For this review, take the finished solid that the model builds, in its own axes (mm). A direction names the side the tool comes from. Give positions to 0.01 mm unless a question says otherwise; leave off trailing zeros. Write each loop counter-clockwise with the first axis right and the second up, starting at its lowest first coordinate (ties: lowest second). Pieces come first, ordered by that corner, then holes. Notation, with made-up numbers: M 34,37.25 L 86,37.25 A17 ccw 86,52.25 Z; hole C -1,44 d9. An arc over 180 degrees is marked long. Write item = value, one per line.
```python
from build123d import *

# Parameters (mm, degrees)
CHAMFER_1_SIZE      = 1
HOLE_WIZARD_M3_1_D  = 3.4
SKETCH_4_R          = 30
CUT_EXTRUDE_1_DEPTH = 8


with BuildPart() as part:
    # 草图1 → 旋转1 (revolve)
    with BuildSketch(Plane(origin=(0, 0, 0), x_dir=(0, 0, -1), z_dir=(1, 0, 0))):
        Polygon((0, 0), (37, 0), (37, 7), (40, 7), (40, 12), (0, 12), align=None)
    revolve(axis=Axis((0, 0, 0), (0, 1, 0)))

    # 倒角1
    chamfer_1_edges = [part.edges().sort_by_distance(p)[0] for p in [
        (0, 0, 37),
    ]]
    chamfer(chamfer_1_edges, length=CHAMFER_1_SIZE)

    # M3 间隙孔1 (through all)
    with Locations(Plane(origin=(0, 12, 0), x_dir=(-1, 0, 0), z_dir=(0, 1, 0))):
        with Locations((0, 25), (-21.650635095, -12.5), (21.650635095, -12.5)):
            Hole(HOLE_WIZARD_M3_1_D / 2)

    # 草图4 → 切除-拉伸1 (cut)
    with BuildSketch(Plane(origin=(0, 12, 0), x_dir=(1, 0, 0), z_dir=(0, 1, 0))):
        with Locations(Location((0, 0, 0), (0, 0, 270))):
            Circle(SKETCH_4_R)
    extrude(amount=-CUT_EXTRUDE_1_DEPTH, mode=Mode.SUBTRACT)


solid = part.part
```
1. Machinability: for faces 4 (the face through (-0.221, 1.972, 26.686)), 5 (the face through (35.4, 7, 11.7)), 6 (the face through (0, 4, 0)), which of the approach directions +Z, -Z, +X, -X, +Y, -Y give a long, thin tool a straight path to every point of the face, cutting with its end or side? Answer none if there is none.
Responses:
face_4 = +Y, -Y
face_5 = -Y
face_6 = +Y
2. The part is to be moulded in two halves that separate along Z. For faces 1 (the face through (19.952, 1.972, -12.425)), 2 (the face through (-30, 12, -6)), 3 (the face through (39.05, 9.54, 8.67)), say which applies: +Z half, -Z half, draft (parallel to the pull), parting line (faces both ways), or undercut.
Responses:
face_1 = undercut
face_2 = draft
face_3 = parting line
3. We need section D-D, the plane y = 9.5. Write out the cut boundary in (x, z).
Responses:
outline = C 0,0 d80; hole C 0,0 d60
4. We need section A-A, the plane x = 0. Write out the cut boundary in (y, z).
Responses:
outline = M 0,-36 L 1,-37 L 7,-37 L 7,-40 L 12,-40 L 12,-30 L 4,-30 L 4,23.3 L 0,23.3 Z; M 0,26.7 L 4,26.7 L 4,30 L 12,30 L 12,40 L 7,40 L 7,37 L 1,37 L 0,36 Z
5. We need section B-B, the plane z = 0. Write out the cut boundary in (x, y), then the cut area to 3 significant figures.
Responses:
outline = M -40,7 L -37,7 L -37,1 L -36,0 L 36,0 L 37,1 L 37,7 L 40,7 L 40,12 L 30,12 L 30,4 L -30,4 L -30,12 L -40,12 Z
area = 437 mm2
6. For line 1 along X through (y, z) = (6.5, 0); line 2 along X through (y, z) = (9.5, 0); line 3 along Y through (x, z) = (-33, 20.5), list the stretches that pass through material, from the lowest coordinate up. Write a range as from..to.
Responses:
line_1 = -37..-30, 30..37
line_2 = -40..-30, 30..40
line_3 = 7..12
7. We need section C-C, the plane y = 2.5. Write out the cut boundary in (x, z).
Responses:
outline = C 0,0 d74; hole C -21.65,-12.5 d3.4; hole C 0,25 d3.4; hole C 21.65,-12.5 d3.4
8. Insertion check: P1, Ø18, axis at x = 9, z = -8, coming from the +Y side; P2, Ø1, axis at x = 22, y = 1.5, coming from the -Z side; P3, Ø1.5, axis at y = 7, z = -1, coming from the +X side. Each pin has a flat end and moves straight along its axis. Give the tip position at first contact, or say it passes through.
Responses:
P1 = 4
P2 = -30.11
P3 = 40
